The listing builds one solid part. Answer for the finished solid, in the listing's coordinates (mm). Coordinates: 2 decimals unless noted, no trailing zeros. One line per item, written item: value. Start each with the question number.
Q1. The part is cut by section A-A on x = 21. Give the number of separate pieces and of enclosed holes in the cut face, then the cut area to 3 significant figures.
Q2. Straight lines are drawn through the part: line 1 along Y through (x, z) = (-15.5, -5.5); line 2 along Y through (x, z) = (-5, -0.5); line 3 along Y through (x, z) = (-17, -8). For each, find the intervals that lie inside material, in ascending order. Write a range as [from, to].
Q3. Each of these flat-tipped pins is pushed along its axis until it touches: pin 1 Ø1.9 at (x, z) = (-1.5, -17.5) entering from +Y; pin 2 Ø8 at (x, y) = (87, 3) entering from +Z; pin 3 Ø8 at (x, z) = (-34.5, -21) entering from -Y; pin 4 Ø10 at (x, y) = (74.5, 8) entering from +Z. Where does it stop, or does it pass through?
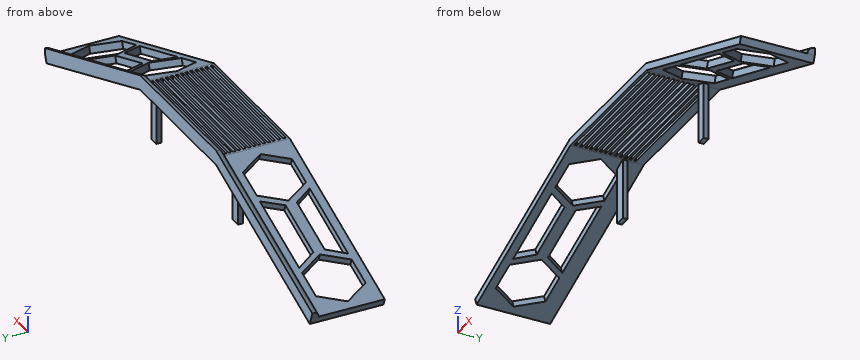
```python
from build123d import *

# Parameters (mm, degrees)
BOSS_EXTRUDE1_DEPTH = 25.4
BOSS_EXTRUDE2_DEPTH = 2.54
FILLET1_R           = 2.54
SKETCH4_W           = 48.892470686
SKETCH4_H           = 0.953754561
SKETCH4_H_2         = 0.953754562
SKETCH4_H_3         = 0.853359345
SKETCH4_H_4         = 0.903556953
SKETCH4_H_5         = 0.853359344
SKETCH4_H_6         = 1.00395217
SKETCH4_H_7         = 1.054149779
CUT_EXTRUDE1_DEPTH  = 4.572
CUT_EXTRUDE2_DEPTH  = 4.572
CUT_EXTRUDE3_DEPTH  = 4.572
SKETCH7_W           = 3.24434763
SKETCH7_H           = 1.675925382
SKETCH7_W_2         = 3.718505185
BOSS_EXTRUDE3_DEPTH = 20.828


with BuildPart() as part:
    # Sketch1 → Boss-Extrude1 (new body)
    with BuildSketch(Plane(origin=(0, 0, 0), x_dir=(1, 0, 0), z_dir=(0, 1, 0))):
        Polygon((0, 0), (50.8, 0), (114.3, 23.790225691), (113.37882382, 26.157298661), (50.8, 2.54), (0, 2.54), (-62.608877976, 26.168775993), (-63.5, 23.790225691), align=None)
    extrude(amount=BOSS_EXTRUDE1_DEPTH)

    # Sketch3 → Boss-Extrude2 (add)
    with BuildSketch(Plane(origin=(0, 25.4, 0), x_dir=(1, 0, 0), z_dir=(0, 1, 0))):
        Polygon((-63.5, 23.790225691), (0, 0), (50.8, 0), (114.3, 23.790225691), (114.3, 21.184727317), (50.8, -2.605498375), (0, -2.605498375), (-64.355998278, 21.505426407), align=None)
    extrude(amount=-BOSS_EXTRUDE2_DEPTH)

    # Fillet1
    # the kernel refuses this fillet: 2.54 mm, written as the material it takes off along each edge
    with BuildSketch(Plane(origin=(5.946375755, 22.86, 4.833303434), x_dir=(0, 1, 0), z_dir=(-0.9364371267563882, 0, -0.35083544238323483))) as fillet1_piece_1_section:
        with BuildLine():
            CenterArc((FILLET1_R, FILLET1_R), FILLET1_R, 180, 90)
            Line((0, FILLET1_R), (0, 0))
            Line((0, 0), (FILLET1_R, 0))
        make_face()
    fillet1_piece_1 = extrude(amount=81.424313079, mode=Mode.PRIVATE)
    fillet1_piece_1 = split(fillet1_piece_1, bisect_by=Plane(origin=(0.305909805, 23.474834282, 0), z_dir=(0, 0, 1)), keep=Keep.TOP, mode=Mode.PRIVATE)
    fillet1_piece_1 = split(fillet1_piece_1, bisect_by=Plane(origin=(0.984368862, 23.474834282, 0.36879303), z_dir=(-0.35083544238323505, 0, 0.9364371267563881)), keep=Keep.TOP, mode=Mode.PRIVATE)
    add(fillet1_piece_1, mode=Mode.SUBTRACT)
    with BuildSketch(Plane(origin=(5.946375755, 22.86, 4.833303434), x_dir=(0, 1, 0), z_dir=(-0.9364371267563882, 0, -0.35083544238323483))) as fillet1_piece_2_section:
        with BuildLine():
            CenterArc((FILLET1_R, FILLET1_R), FILLET1_R, 180, 90)
            Line((0, FILLET1_R), (0, 0))
            Line((0, 0), (FILLET1_R, 0))
        make_face()
    fillet1_piece_2 = extrude(amount=81.424313079, mode=Mode.PRIVATE)
    fillet1_piece_2 = split(fillet1_piece_2, bisect_by=Plane(origin=(3.480294326, 22.834935374, 0), z_dir=(0, 0, 1)), keep=Keep.TOP, mode=Mode.PRIVATE)
    fillet1_piece_2 = split(fillet1_piece_2, bisect_by=Plane(origin=(3.46295466, 22.834935374, 1.297393274), z_dir=(0.35083544238323505, 0, -0.9364371267563881)), keep=Keep.TOP, mode=Mode.PRIVATE)
    add(fillet1_piece_2, mode=Mode.SUBTRACT)
    with BuildSketch(Plane(origin=(5.946375755, 22.86, 4.833303434), x_dir=(0, 1, 0), z_dir=(-0.9364371267563882, 0, -0.35083544238323483))) as fillet1_piece_3_section:
        with BuildLine():
            CenterArc((FILLET1_R, FILLET1_R), FILLET1_R, 180, 90)
            Line((0, FILLET1_R), (0, 0))
            Line((0, 0), (FILLET1_R, 0))
        make_face()
    fillet1_piece_3 = extrude(amount=81.424313079, mode=Mode.PRIVATE)
    fillet1_piece_3 = split(fillet1_piece_3, bisect_by=Plane(origin=(-37.699790788, 23.430211039, 0), z_dir=(0, 0, -1)), keep=Keep.TOP, mode=Mode.PRIVATE)
    fillet1_piece_3 = split(fillet1_piece_3, bisect_by=Plane(origin=(-37.047344153, 23.430211039, -13.879758719), z_dir=(-0.35083544238323505, 0, 0.9364371267563881)), keep=Keep.TOP, mode=Mode.PRIVATE)
    add(fillet1_piece_3, mode=Mode.SUBTRACT)
    with BuildSketch(Plane(origin=(57.15, 22.86, 2.605498375), x_dir=(0, 1, 0), z_dir=(-1, 0, 0))) as fillet1_piece_4:
        with BuildLine():
            CenterArc((FILLET1_R, FILLET1_R), FILLET1_R, 180, 90)
            Line((0, FILLET1_R), (0, 0))
            Line((0, 0), (FILLET1_R, 0))
        make_face()
    extrude(amount=63.5, mode=Mode.SUBTRACT)
    with BuildSketch(Plane(origin=(120.246375755, 22.86, -23.412532376), x_dir=(0, 1, 0), z_dir=(-0.9364371267563881, 0, 0.3508354423832351))) as fillet1_piece_5_section:
        with BuildLine():
            CenterArc((FILLET1_R, FILLET1_R), FILLET1_R, 180, 90)
            Line((0, FILLET1_R), (0, 0))
            Line((0, 0), (FILLET1_R, 0))
        make_face()
    fillet1_piece_5 = extrude(amount=80.510211904, mode=Mode.PRIVATE)
    fillet1_piece_5 = split(fillet1_piece_5, bisect_by=Plane(origin=(88.071552379, 23.43012107, 0), z_dir=(0, 0, -1)), keep=Keep.TOP, mode=Mode.PRIVATE)
    fillet1_piece_5 = split(fillet1_piece_5, bisect_by=Plane(origin=(87.41915819, 23.43012107, -13.719339181), z_dir=(0.35083544238323505, 0, 0.9364371267563881)), keep=Keep.TOP, mode=Mode.PRIVATE)
    add(fillet1_piece_5, mode=Mode.SUBTRACT)
    with BuildSketch(Plane(origin=(120.246375755, 22.86, -23.412532376), x_dir=(0, 1, 0), z_dir=(-0.9364371267563881, 0, 0.3508354423832351))) as fillet1_piece_6_section:
        with BuildLine():
            CenterArc((FILLET1_R, FILLET1_R), FILLET1_R, 180, 90)
            Line((0, FILLET1_R), (0, 0))
            Line((0, 0), (FILLET1_R, 0))
        make_face()
    fillet1_piece_6 = extrude(amount=80.510211904, mode=Mode.PRIVATE)
    fillet1_piece_6 = split(fillet1_piece_6, bisect_by=Plane(origin=(50.494090195, 23.474834282, 0), z_dir=(0, 0, 1)), keep=Keep.TOP, mode=Mode.PRIVATE)
    fillet1_piece_6 = split(fillet1_piece_6, bisect_by=Plane(origin=(49.815631138, 23.474834282, 0.36879303), z_dir=(0.35083544238323505, 0, 0.9364371267563881)), keep=Keep.TOP, mode=Mode.PRIVATE)
    add(fillet1_piece_6, mode=Mode.SUBTRACT)
    with BuildSketch(Plane(origin=(120.246375755, 22.86, -23.412532376), x_dir=(0, 1, 0), z_dir=(-0.9364371267563881, 0, 0.3508354423832351))) as fillet1_piece_7_section:
        with BuildLine():
            CenterArc((FILLET1_R, FILLET1_R), FILLET1_R, 180, 90)
            Line((0, FILLET1_R), (0, 0))
            Line((0, 0), (FILLET1_R, 0))
        make_face()
    fillet1_piece_7 = extrude(amount=80.510211904, mode=Mode.PRIVATE)
    fillet1_piece_7 = split(fillet1_piece_7, bisect_by=Plane(origin=(47.319705674, 22.834935374, 0), z_dir=(0, 0, 1)), keep=Keep.TOP, mode=Mode.PRIVATE)
    fillet1_piece_7 = split(fillet1_piece_7, bisect_by=Plane(origin=(47.33704534, 22.834935374, 1.297393274), z_dir=(-0.35083544238323505, 0, -0.9364371267563881)), keep=Keep.TOP, mode=Mode.PRIVATE)
    add(fillet1_piece_7, mode=Mode.SUBTRACT)

    # Sketch4 → Cut-Extrude1 (cut)
    with BuildSketch(Plane.XY):
        with Locations((25.43082689, 1.319550291)):
            Rectangle(SKETCH4_W, SKETCH4_H)
        with Locations((25.43082689, 3.126664197)):
            Rectangle(SKETCH4_W, SKETCH4_H_2)
        with Locations((25.43082689, 4.883580495)):
            Rectangle(SKETCH4_W, SKETCH4_H_3)
        with Locations((25.43082689, 6.590299184)):
            Rectangle(SKETCH4_W, SKETCH4_H_2)
        with Locations((25.43082689, 8.271919069)):
            Rectangle(SKETCH4_W, SKETCH4_H_4)
        with Locations((25.43082689, 9.978637758)):
            Rectangle(SKETCH4_W, SKETCH4_H_4)
        with Locations((25.43082689, 11.559862426)):
            Rectangle(SKETCH4_W, SKETCH4_H_5)
        with Locations((25.43082689, 13.29167992)):
            Rectangle(SKETCH4_W, SKETCH4_H_6)
        with Locations((25.43082689, 15.073695022)):
            Rectangle(SKETCH4_W, SKETCH4_H_7)
        with Locations((25.43082689, 16.83061132)):
            Rectangle(SKETCH4_W, SKETCH4_H)
        with Locations((25.43082689, 18.562428813)):
            Rectangle(SKETCH4_W, SKETCH4_H_6)
        with Locations((25.43082689, 20.168752286)):
            Rectangle(SKETCH4_W, SKETCH4_H_4)
        with Locations((25.43082689, 21.800174562)):
            Rectangle(SKETCH4_W, SKETCH4_H_3)
    extrude(amount=-CUT_EXTRUDE1_DEPTH, mode=Mode.SUBTRACT)

    # Sketch5 → Cut-Extrude2 (cut)
    with BuildSketch(Plane(origin=(6.252743788, 0, 16.689594948), x_dir=(0.9364371267563881, 0, -0.35083544238323516), z_dir=(0.35083544238323516, 0, 0.9364371267563881))):
        Polygon((95.385492335, 2.513306314), (91.342188498, 9.687056546), (71.771776783, 9.687056546), (67.681786758, 2.513306314), align=None)
        Polygon((107.872330044, 2.586895642), (112.935981689, 11.50457622), (107.744869589, 20.34866747), (97.490105842, 20.275078142), (92.426454197, 11.357397564), (97.617566297, 2.513306314), align=None)
        Polygon((65.396301526, 2.513306314), (70.556591706, 11.410782697), (65.431296219, 20.328463275), (55.145710553, 20.34866747), (49.985420372, 11.451191088), (55.110715859, 2.53351051), align=None)
        Polygon((91.342188498, 12.895099362), (71.771776783, 12.895099362), (67.681786758, 20.328463275), (95.385492335, 20.328463275), align=None)
    extrude(amount=-CUT_EXTRUDE2_DEPTH, mode=Mode.SUBTRACT)

    # Sketch6 → Cut-Extrude3 (cut)
    with BuildSketch(Plane(origin=(0, 0, 0), x_dir=(0.9364371267563881, 0, 0.35083544238323516), z_dir=(-0.35083544238323516, 0, 0.9364371267563881))):
        Polygon((-20.081392491, 2.871915117), (-47.639225338, 2.871915117), (-43.82197308, 9.151723276), (-23.965625147, 9.151723276), align=None)
        Polygon((-7.714681248, 2.947668713), (-2.860571572, 11.506740488), (-7.845890325, 19.990058667), (-17.685318752, 19.914305072), (-22.539428428, 11.355233297), (-17.554109675, 2.871915117), align=None)
        Polygon((-50.125492855, 2.871915117), (-45.20547879, 11.468344332), (-50.190197838, 20.027416107), (-60.094930953, 19.990058667), (-65.014945018, 11.393629453), (-60.030225969, 2.834557678), align=None)
        Polygon((-23.965625147, 13.042600451), (-43.82197308, 13.042600451), (-48.142272105, 20.027416107), (-20.081392491, 20.027416107), align=None)
    extrude(amount=-CUT_EXTRUDE3_DEPTH, mode=Mode.SUBTRACT)

    # Sketch7 → Boss-Extrude3 (add)
    with BuildSketch(Plane(origin=(0, 0, -2.54), x_dir=(-1, 0, 0), z_dir=(0, 0, -1))):
        with Locations((-52.422173815, 18.963924101)):
            Rectangle(SKETCH7_W, SKETCH7_H)
        with Locations((1.859252593, 18.963924101)):
            Rectangle(SKETCH7_W_2, SKETCH7_H)
    extrude(amount=BOSS_EXTRUDE3_DEPTH)


solid = part.part
```
Output:
1. separate pieces: 14
1. enclosed holes: 0
1. area: 38.9 mm^2
2. line 1: y = [22.89, 25.4]
2. line 2: y = [23.27, 25.4]
2. line 3: y = [0, 4.87], [18.08, 25.4]
3. pin 1: stops at y = 19.8
3. pin 2: stops at z = -12.07
3. pin 3: passes through
3. pin 4: stops at z = -7.08
